```python
from build123d import *

# Parameters (mm, degrees)
SKETCH2_R           = 19.05
BOSS_EXTRUDE1_DEPTH = 12.7
SKETCH2_5_R         = 25.4
SKETCH2_5_R_2       = 19.05
BOSS_EXTRUDE3_DEPTH = 38.1
SHELL2_T            = -2.54
SKETCH32_R          = 9.525
CUT_EXTRUDE1_DEPTH  = 50.8
SKETCH2_10_R        = 25.4
SKETCH2_10_R_2      = 19.05
BOSS_EXTRUDE4_DEPTH = 2.54


with BuildPart() as part:
    # Sketch2 → Boss-Extrude1 (new body)
    with BuildSketch(Plane(origin=(0, 0, 0), x_dir=(1, 0, 0), z_dir=(0, 1, 0))):
        with Locations(Location((0, 0, 0), (0, 0, 270))):
            Circle(SKETCH2_R)
    extrude(amount=BOSS_EXTRUDE1_DEPTH)

    # Shell2
    shell2_openings = [part.faces().sort_by_distance(p)[0] for p in [
        (0, 12.7, 0),
        (0, 0, 0),
    ]]
    offset(amount=SHELL2_T, openings=shell2_openings, kind=Kind.INTERSECTION)



with BuildPart() as body_2:
    # Sketch2_5 → Boss-Extrude3 (new body)
    with BuildSketch(Plane(origin=(0, 0, 0), x_dir=(1, 0, 0), z_dir=(0, 1, 0))):
        with Locations(Location((0, 0, 0), (0, 0, 270))):
            Circle(SKETCH2_5_R)
        with Locations(Location((0, 0, 0), (0, 0, 270))):
            Circle(SKETCH2_5_R_2, mode=Mode.SUBTRACT)
    extrude(amount=-BOSS_EXTRUDE3_DEPTH)

    # Sketch32 → Cut-Extrude1 (cut)
    with BuildSketch(Plane(origin=(0, 0, 0), x_dir=(0, 0, -1), z_dir=(1, 0, 0))):
        with Locations((0, -19.05)):
            Circle(SKETCH32_R)
    extrude(amount=-CUT_EXTRUDE1_DEPTH, mode=Mode.SUBTRACT)


with BuildPart() as part_1:
    add(part.part)

    add(body_2.part)  # Boss-Extrude4 merges body 2
    # Sketch2_10 → Boss-Extrude4 (add)
    with BuildSketch(Plane(origin=(0, 0, 0), x_dir=(1, 0, 0), z_dir=(0, 1, 0))):
        with Locations(Location((0, 0, 0), (0, 0, 270))):
            Circle(SKETCH2_10_R)
        with Locations(Location((0, 0, 0), (0, 0, 270))):
            Circle(SKETCH2_10_R_2, mode=Mode.SUBTRACT)
    extrude(amount=BOSS_EXTRUDE4_DEPTH)


solid = part_1.part
```
Input: part model. Units: mm. Frame: model coordinates. A direction names the side the tool comes from. Give positions to 0.01 mm unless a question says otherwise; leave off trailing zeros. Order: outer loops, then holes, each group sorted by start corner. A loop starts at its lowest first (then second) coordinate and runs counter-clockwise, first axis right, second up. Notation, with made-up numbers: (72.5, 81.5) - (91.5, 81.5) arc R10 ccw to (91.5, 89.5) - close; hole circle Ø3 at (42, -36). An arc over 180 degrees is marked (long way). Put each result on its own line as item: value.
Item 1: Draft query along Y for faces 1 (the cylindrical face through (-11.59, 7.55, -15.12)), 2 (the cylindrical face through (-20.9, -22.7, -8.8)), 3 (the flat face through (19, 2.54, 4)), 4 (the flat face through (19, -38.1, 4)). Return one class per face: +Y half, -Y half, draft (parallel to the pull), parting line (faces both ways), or undercut.
Found:
face 1: draft
face 2: undercut
face 3: +Y half
face 4: -Y half
Item 2: Section query D-D, the plane z = -12. Return loops of the section in (x, y), then the cut area to 3 significant figures.
Found:
outline: (-22.39, -38.1) - (-14.8, -38.1) - (-14.8, 0) - (-11.34, 0) - (-11.34, 12.7) - (-14.8, 12.7) - (-14.8, 2.54) - (-22.39, 2.54) - close; (11.34, 0) - (14.8, 0) - (14.8, -38.1) - (22.39, -38.1) - (22.39, 2.54) - (14.8, 2.54) - (14.8, 12.7) - (11.34, 12.7) - close
area: 705 mm^2
Item 3: Contact query for flat-ended pins moving along their axis: pin 1 (2 mm diameter, centred on y = -8, z = -8.5, fed in from +X); pin 2 (1 mm diameter, centred on x = 2.5, y = -31.5, fed in from +Z); pin 3 (1.5 mm diameter, centred on x = 0.5, y = 6.5, fed in from -Z). Output: stop coordinate, or through.
Found:
pin 1: stops at x = 24.27
pin 2: stops at z = 25.32
pin 3: stops at z = -19.05
Item 4: Ray query, L1, parallel to X at y = 9.75, z = 0; L2, parallel to Y at x = -21, z = 0 (3 decimals); L3, parallel to Y at x = 12.5, z = 20. Return the intervals inside material, ascending. Write a range as from..to.
Found:
L1: x = -19.05..-16.51, 16.51..19.05
L2: y = -38.1..-28.575, -9.525..2.54
L3: y = -38.1..2.54
Item 5: Section query C-C, the plane y = -31. Return loops of the section in (x, z).
Found:
outline: circle Ø50.8 at (0, 0); hole circle Ø38.1 at (0, 0)
Item 6: Section query A-A, the plane z = 0. Return loops of the section in (x, y) (3 decimals).
Found:
outline: (-25.4, -38.1) - (-19.05, -38.1) - (-19.05, -28.575) - (-25.4, -28.575) - close; (-25.4, -9.525) - (-19.05, -9.525) - (-19.05, 0) - (-16.51, 0) - (-16.51, 12.7) - (-19.05, 12.7) - (-19.05, 2.54) - (-25.4, 2.54) - close; (16.51, 0) - (19.05, 0) - (19.05, -38.1) - (25.4, -38.1) - (25.4, 2.54) - (19.05, 2.54) - (19.05, 12.7) - (16.51, 12.7) - close
Item 7: Section query B-B, the plane x = 0. Return loops of the section in (y, z), then the cut area to 3 significant figures.
Found:
outline: (-38.1, -25.4) - (2.54, -25.4) - (2.54, -19.05) - (12.7, -19.05) - (12.7, -16.51) - (0, -16.51) - (0, -19.05) - (-38.1, -19.05) - close; (-38.1, 19.05) - (0, 19.05) - (0, 16.51) - (12.7, 16.51) - (12.7, 19.05) - (2.54, 19.05) - (2.54, 25.4) - (-38.1, 25.4) - close
area: 581 mm^2
Item 8: Access query for faces 5 (the cylindrical face through (18.888, -18.783, -2.48)), 6 (the cylindrical face through (-10.05, 6.26, -13.1)). Directions: +Z, -Z, +X, -X, +Y, -Y. A direction counts if a zero-diameter tool reaches every point of the face in a straight line with its end or side. Return the directions, or none.
Found:
face 5: -Y
face 6: +Y, -Y
